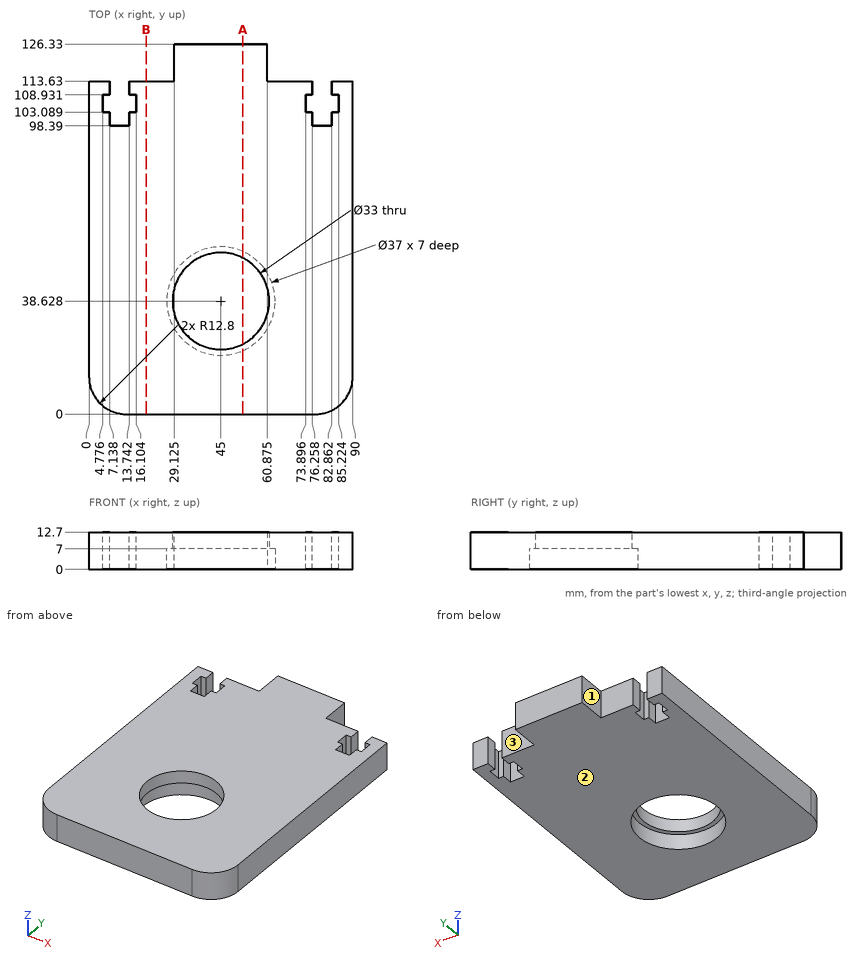
Answer from the drawing. Dimensions are ordinates in mm from the lowest x, y and z of the part. A direction names the side the tool comes from. Give positions to 0.01 mm unless a question says otherwise; leave off trailing zeros. Order: outer loops, then holes, each group sorted by start corner. A loop starts at its lowest first (then second) coordinate and runs counter-clockwise, first axis right, second up. Notation, with made-up numbers: (68, 74.25) - (122, 74.25) arc R35 cw to (122, 110.25) - close; hole circle Ø7 at (23, 49.5). An arc over 180 degrees is marked (long way). One line per item, written item: value. Start each with the question number.
1) A tool of negligible diameter and unlimited length cuts with its end or side. For the marked faces 1, 2 and 3, from which of +Z, -Z, +X, -X, +Y, -Y can it reach the whole face along a straight path? Write none if from no direction.
2) Find the intervals of material crossed by L1, parallel to X at y = 109, z = 2.25; L2, parallel to Y at x = 45, z = 9.55; L3, parallel to Y at x = 45, z = 4, in increasing order.
3) A cutting plane is placed at A-A on x = 52.5. Give the vertices of the cut face in (y, z) (1 decimal).
4) Given pin 1 Ø1 at (x, z) = (20, 11.5) entering from +Y; pin 2 Ø1 at (x, z) = (79, 9.5) entering from +Y; pin 3 Ø4 at (x, y) = (55.5, 51) entering from -Z, each flat-ended and moving along its own axis, determine where each tip first touches the part or whether it passes through.
5) A cutting plane is placed at B-B on x = 19.5. Give the vertices of the cut face in (y, z).
Answer sheet:
1. face 1: +Z, -Z, -X, +Y
1. face 2: -Z, +X, -X, +Y, -Y
1. face 3: +Z, -Z, +X, +Y
2. L1: x = 0 to 7.14, 13.74 to 76.26, 82.86 to 90
2. L2: y = 0 to 22.13, 55.13 to 126.33
2. L3: y = 0 to 20.13, 57.13 to 126.33
3. outline: (0, 0) - (21.7, 0) - (21.7, 7) - (23.9, 7) - (23.9, 12.7) - (0, 12.7) - close; (53.3, 7) - (55.5, 7) - (55.5, 0) - (126.3, 0) - (126.3, 12.7) - (53.3, 12.7) - close
4. pin 1: stops at y = 113.63
4. pin 2: stops at y = 98.39
4. pin 3: stops at z = 7
5. outline: (0, 0) - (113.63, 0) - (113.63, 12.7) - (0, 12.7) - close
